The drawing under review shows one solid part. Ordinate dimensions are in mm from its lowest x, y, z. Round coordinates to 2 decimals unless told otherwise and drop trailing zeros. Order: outer loops, then holes, each group sorted by start corner. A loop starts at its lowest first (then second) coordinate and runs counter-clockwise, first axis right, second up. Notation, with made-up numbers: M 32.5,26.25 L 75.5,26.25 A11 cw 75.5,45.25 Z; hole C -2,-31 d4. An arc over 180 degrees is marked long. Answer as a JSON object with one key per item and string values. Group by question number.
1) Consider section B-B, the plane z = 1.5. Write out the cut boundary in (x, y).
2) Consider section C-C, the plane y = 56.6. Write out the cut boundary in (x, z), then the cut area to 3 significant figures.
3) Consider section D-D, the plane x = 52. Write out the cut boundary in (y, z).
4) Insertion check: pin 1 Ø6.5 at (x, y) = (52, 12.2) entering from +Z. The pin has a flat end and moves straight along its axis. Give the tip position at first contact, or say it passes through.
5) Consider section A-A, the plane x = 19. Write out the cut boundary in (y, z), then the cut area to 3 significant figures.
6) To check wall thickness, follow line 1 (X direction, y = 12.2, z = 3.25); line 2 (X direction, y = 34.4, z = 5); line 3 (Y direction, x = 52, z = 3). State the ranges of each line that lie inside material, in increasing order.
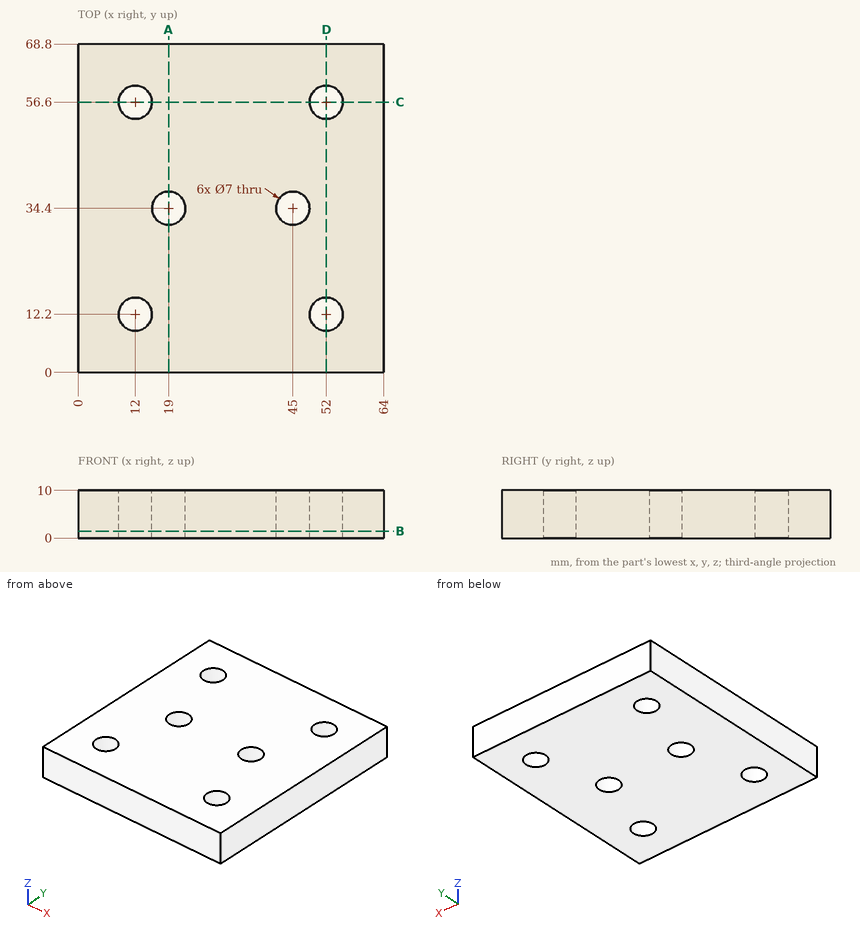
Results list:
{
 "1": {"outline": "M 0,0 L 64,0 L 64,68.8 L 0,68.8 Z; hole C 12,12.2 d7; hole C 12,56.6 d7; hole C 19,34.4 d7; hole C 45,34.4 d7; hole C 52,12.2 d7; hole C 52,56.6 d7"},
 "2": {"outline": "M 0,0 L 8.5,0 L 8.5,10 L 0,10 Z; M 15.5,0 L 48.5,0 L 48.5,10 L 15.5,10 Z; M 55.5,0 L 64,0 L 64,10 L 55.5,10 Z", "area": "500 mm^2"},
 "3": {"outline": "M 0,0 L 8.7,0 L 8.7,10 L 0,10 Z; M 15.7,0 L 53.1,0 L 53.1,10 L 15.7,10 Z; M 60.1,0 L 68.8,0 L 68.8,10 L 60.1,10 Z"},
 "4": {"pin 1": "through"},
 "5": {"outline": "M 0,0 L 30.9,0 L 30.9,10 L 0,10 Z; M 37.9,0 L 68.8,0 L 68.8,10 L 37.9,10 Z", "area": "618 mm^2"},
 "6": {"line 1": "0 to 8.5, 15.5 to 48.5, 55.5 to 64", "line 2": "0 to 15.5, 22.5 to 41.5, 48.5 to 64", "line 3": "0 to 8.7, 15.7 to 53.1, 60.1 to 68.8"}
}
